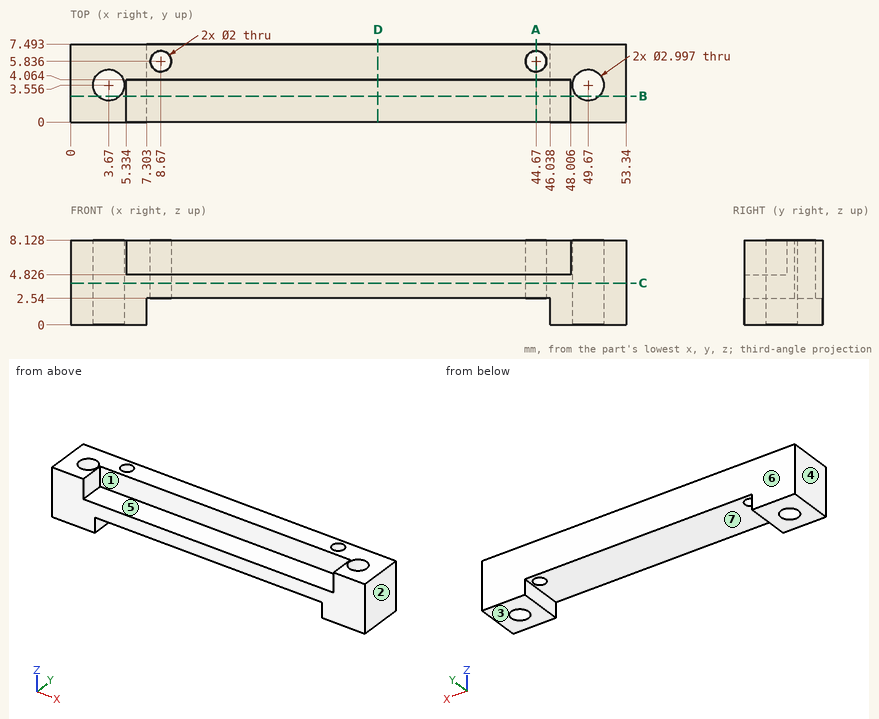
Print and shaded views of the part. All mm, measured from the part's lowest x, y and z. A direction names the side the tool comes from. Coordinates: 2 decimals unless noted, no trailing zeros. Loops run counter-clockwise (first coordinate to the right, second up) from the corner with the lowest first, then second, coordinate; pieces in that order, holes last. Notation, with made-up numbers: (-10, 77.5) -> (31, 77.5) arc R22 cw to (31, 93.5) -> close; hole circle Ø3 at (-23, 63). An arc over 180 degrees is marked (long way). Use one line per item in the form item = value. Start each with the question number.
(1) Cut at C-C on z = 4. Give the cut face in (x, y) (1 decimal), and give its area (3 significant figures).
(2) Cut at A-A on x = 44.67. Give the cut face in (y, z) (1 decimal).
(3) Tool access for the marked faces 5, 6 and 7: list every direction of +Z, -Z, +X, -X, +Y, -Y with a clear straight run to the whole face (end or side of a thin tool).
(4) Probe probe 1 along X at (y, z) = (3.5, 1.25); probe 2 along X at (y, z) = (4, 6.5) (1 decimal); probe 3 along Y at (x, z) = (8.67, 3.8) (1 decimal). List the from-to ranges inside material, lowest first. Write a range as from..to.
(5) Pull direction X, two halves, no side cores. Call the marked faces 1, 2, 3 and 4: pulls with the +X half, pulls with the -X half, needs draft (parallel to the pull), parting line crosses it, or undercut.
(6) Cut at B-B on y = 2.5. Give the cut face in (x, z) (1 decimal).
(7) Cut at D-D on x = 29.5. Give the cut face in (y, z) (1 decimal).
(8) Flat gauge pins, fed straight in: pin 1 (3.5 mm diameter, centred on x = 35.5, y = 5, fed in from -Z); pin 2 (2.5 mm diameter, centred on x = 29, z = 6.5, fed in from -Y); pin 3 (1.8 mm diameter, centred on x = 8.67, y = 5.84, fed in from +Z); pin 4 (3.5 mm diameter, centred on x = 29, y = 2, fed in from +Z). Where does each tip first touch, or does it go through?
Values:
q1.outline = (0, 0) -> (53.3, 0) -> (53.3, 7.5) -> (0, 7.5) -> close; hole circle Ø3 at (3.7, 3.6); hole circle Ø2 at (8.7, 5.8); hole circle Ø2 at (44.7, 5.8); hole circle Ø3 at (49.7, 3.6)
q1.area = 379 mm2
q2.outline = (0, 2.5) -> (4.8, 2.5) -> (4.8, 8.1) -> (4.1, 8.1) -> (4.1, 4.8) -> (0, 4.8) -> close; (6.8, 2.5) -> (7.5, 2.5) -> (7.5, 8.1) -> (6.8, 8.1) -> close
q3.face_5 = +Z, -Y
q3.face_6 = +Z, -Z, +X, -X, +Y
q3.face_7 = -Z, +Y, -Y
q4.probe_1 = 0..2.17, 5.17..7.3, 46.04..48.17, 51.17..53.34
q4.probe_2 = 0..2.2, 5.1..5.3, 48..48.2, 51.1..53.3
q4.probe_3 = 0..4.8, 6.8..7.5
q5.face_1 = undercut
q5.face_2 = pulls with the +X half
q5.face_3 = needs draft
q5.face_4 = pulls with the -X half
q6.outline = (0, 0) -> (2.6, 0) -> (2.6, 8.1) -> (0, 8.1) -> close; (4.7, 0) -> (7.3, 0) -> (7.3, 2.5) -> (46, 2.5) -> (46, 0) -> (48.6, 0) -> (48.6, 8.1) -> (48, 8.1) -> (48, 4.8) -> (5.3, 4.8) -> (5.3, 8.1) -> (4.7, 8.1) -> close; (50.7, 0) -> (53.3, 0) -> (53.3, 8.1) -> (50.7, 8.1) -> close
q7.outline = (0, 2.5) -> (7.5, 2.5) -> (7.5, 8.1) -> (4.1, 8.1) -> (4.1, 4.8) -> (0, 4.8) -> close
q8.pin_1 = 2.54
q8.pin_2 = 4.06
q8.pin_3 = through
q8.pin_4 = 4.83
